Work out the finished part from the listing and answer in its coordinate system (mm). A direction names the side the tool comes from. Give positions to 0.01 mm unless a question says otherwise; leave off trailing zeros. Loops run counter-clockwise (first coordinate to the right, second up) from the corner with the lowest first, then second, coordinate; pieces in that order, holes last.
```python
from build123d import *

# Parameters (mm, degrees)
SKETCH1_W            = 18.542
SKETCH1_H            = 17.78
BOSS_EXTRUDE4_DEPTH  = 1.27
SKETCH4_W            = 18.542
SKETCH4_H            = 17.78
BOSS_EXTRUDE5_DEPTH  = 1.27
BOSS_EXTRUDE6_DEPTH  = 18.542
SKETCH7_W            = 11.43
SKETCH7_H            = 10.16
BOSS_EXTRUDE7_DEPTH  = 1.27
SKETCH12_W           = 12.7
SKETCH12_H           = 12.7
BOSS_EXTRUDE11_DEPTH = 2.286
CUT_EXTRUDE2_DEPTH   = 23.616343139
BOSS_EXTRUDE12_DEPTH = 1.27


with BuildPart() as part:
    # Sketch1 → Boss-Extrude4 (new body)
    with BuildSketch(Plane.XY):
        Rectangle(SKETCH1_W, SKETCH1_H)
    extrude(amount=-BOSS_EXTRUDE4_DEPTH)



with BuildPart() as body_2:
    # Sketch4 → Boss-Extrude5 (new body)
    with BuildSketch(Plane.XY.offset(-13.97)):
        Rectangle(SKETCH4_W, SKETCH4_H)
    extrude(amount=BOSS_EXTRUDE5_DEPTH)


with BuildPart() as part_1:
    add(part.part)

    add(body_2.part)  # Boss-Extrude6 merges body 2
    # Sketch6 → Boss-Extrude6 (add)
    with BuildSketch(Plane.ZY.offset(9.271)):
        with BuildLine():
            Line((-13.97, 8.89), (-12.7, 8.89))
            ThreePointArc((-12.7, 8.89), (-6.985, 14.605), (-1.27, 8.89))
            Line((-1.27, 8.89), (0, 8.89))
            ThreePointArc((0, 8.89), (-6.985, 15.875), (-13.97, 8.89))
        make_face()
    extrude(amount=-BOSS_EXTRUDE6_DEPTH)

    # Sketch7 → Boss-Extrude7 (add)
    with BuildSketch(Plane.ZY.offset(9.271)):
        with Locations((-6.985, -3.81)):
            Rectangle(SKETCH7_W, SKETCH7_H)
    extrude(amount=-BOSS_EXTRUDE7_DEPTH)

    # Sketch12 → Boss-Extrude11 (add)
    with BuildSketch(Plane(origin=(0, 0, -13.97), x_dir=(-1, 0, 0), z_dir=(0, 0, -1))):
        with Locations((0, -2.54)):
            Rectangle(SKETCH12_W, SKETCH12_H)
    extrude(amount=BOSS_EXTRUDE11_DEPTH)

    # Sketch13 → Cut-Extrude2 (cut, through all)
    with BuildSketch(Plane(origin=(0, 3.81, 0), x_dir=(1, 0, 0), z_dir=(0, 1, 0))):
        Polygon((-5.08, 13.97), (5.08, 13.97), (5.08, 15.493275397), (-5.08, 15.748), align=None)
    extrude(amount=-CUT_EXTRUDE2_DEPTH, mode=Mode.SUBTRACT)

    # Sketch8 → Boss-Extrude12 (add)
    with BuildSketch(Plane(origin=(9.271, 0, 0), x_dir=(0, 0, -1), z_dir=(1, 0, 0))):
        Polygon((1.905, 1.27), (1.27, 1.27), (1.27, -8.89), (12.7, -8.89), (12.7, 1.27), (10.795, 1.27), align=None)
    extrude(amount=-BOSS_EXTRUDE12_DEPTH)


solid = part_1.part
```
Q1. Section C-C on x = 3.75 is taken. Give the vertices of the cut face in (y, z) (3 decimals).
Q2. Which of the six approach directions +Z, -Z, +X, -X, +Y, -Y give full straight-line access (tool end or side, diameter ignored) to faces 5 (the face through (-6.35, -3, -15)), 6 (the face through (0, 3.81, -16)), 7 (the face through (8.001, -4, -7)), 8 (the face through (-9, 1.27, -7))?
Q3. Section D-D on x = 0.25 is taken. Give the vertices of the cut face in (y, z) (3 decimals), plus the area to 3 significant figures.
Q4. Section B-B on y = -6.75 is taken. Give the vertices of the cut face in (x, z).
Q5. Determine the mould class of faces 1 (the face through (6.35, -3, -15)), 2 (the face through (-0.13, 14.604, -7.111)), 3 (the face through (-5.08, -2, -15)), 4 (the face through (-9.271, 1, -7)) for opening direction X: +X half, -X half, draft (parallel to the pull), parting line (faces both ways), or undercut.
Q6. Given pin 1 (2.5 mm diameter, centred on y = -3, z = -15, fed in from +X); pin 2 (0.7 mm diameter, centred on y = -5.5, z = -15.5, fed in from -X); pin 3 (0.6 mm diameter, centred on x = 9, z = -7.5, fed in from +Y); pin 4 (3 mm diameter, centred on y = 6, z = -10.5, fed in from +X), each flat-ended and moving along its own axis, determine where each tip first touches the part or whether it passes through.
Q7. Section A-A on y = 7 is taken. Give the vertices of the cut face in (x, z), plus the area to 3 significant figures.
Q8. Consider line 1 along Z through (x, y) = (7, 1.5); line 2 along X through (y, z) = (0.75, -12); line 3 along Z through (x, y) = (-3.25, -6.75). Determine where each line is inside the solid, lowest interval first.
Check result:
1. outline: (-8.89, -16.256) - (3.81, -16.256) - (3.81, -15.527) - (-8.89, -15.527) - close; (-8.89, -13.97) - (8.89, -13.97) arc R6.985 ccw to (8.89, 0) - (-8.89, 0) - (-8.89, -1.27) - (8.89, -1.27) arc R5.715 cw to (8.89, -12.7) - (-8.89, -12.7) - close
2. face 5: -Z, -X, +Y, -Y
2. face 6: -Z, +X, -X, +Y
2. face 7: -Y
2. face 8: +X, -X
3. outline: (-8.89, -16.256) - (3.81, -16.256) - (3.81, -15.614) - (-8.89, -15.614) - close; (-8.89, -13.97) - (8.89, -13.97) arc R6.985 ccw to (8.89, 0) - (-8.89, 0) - (-8.89, -1.27) - (8.89, -1.27) arc R5.715 cw to (8.89, -12.7) - (-8.89, -12.7) - close
3. area: 78.6 mm2
4. outline: (-9.27, -13.97) - (-6.35, -13.97) - (-6.35, -16.26) - (6.35, -16.26) - (6.35, -13.97) - (9.27, -13.97) - (9.27, 0) - (-9.27, 0) - close; hole (-8, -12.7) - (8, -12.7) - (8, -1.27) - (-8, -1.27) - close; hole (-5.08, -15.75) - (5.08, -15.49) - (5.08, -13.97) - (-5.08, -13.97) - close
5. face 1: +X half
5. face 2: draft
5. face 3: undercut
5. face 4: -X half
6. pin 1: stops at x = 9.27
6. pin 2: stops at x = -6.35
6. pin 3: stops at y = 15.87
6. pin 4: passes through
7. outline: (-9.27, -13.97) - (9.27, -13.97) - (9.27, -12.7) - (-9.27, -12.7) - close; (-9.27, -1.27) - (9.27, -1.27) - (9.27, 0) - (-9.27, 0) - close
7. area: 47.1 mm2
8. line 1: z = -13.97 to -12.7, -1.27 to 0
8. line 2: x = -9.27 to -8, 8 to 9.27
8. line 3: z = -16.26 to -15.7, -13.97 to -12.7, -1.27 to 0
